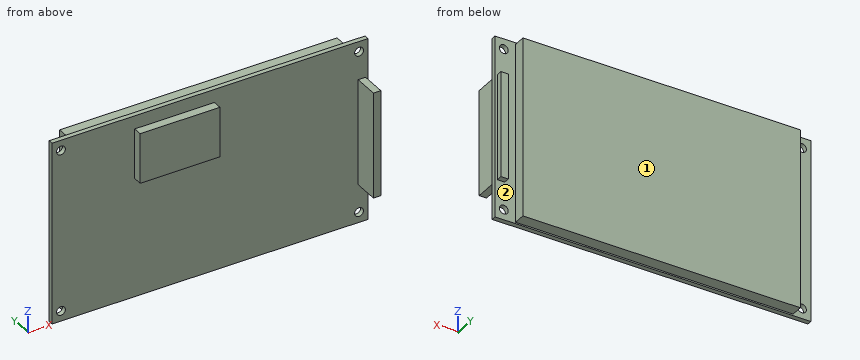
from build123d import *

# Parameters (mm, degrees)
SCHIZZO1_W                        = 94
SCHIZZO1_H                        = 61
ESTRUSIONE_ESTRUSIONE1_DEPTH      = 4
SCHIZZO2_W                        = 107
SCHIZZO2_H                        = 62
ESTRUSIONE_ESTRUSIONE2_DEPTH      = 1.6
ESTRUSIONE_ESTRUSIONE3_DEPTH      = 2
ESTRUSIONE_ESTRUSIONE3_DEPTH_BACK = 10
SCHIZZO4_W                        = 2.5
SCHIZZO4_H                        = 36
SCHIZZO6_R                        = 1.5
TAGLIO_ESTRUSIONE1_DEPTH          = 2
SCHIZZO7_W                        = 27
SCHIZZO7_H                        = 17
ESTRUSIONE_ESTRUSIONE4_DEPTH      = 3


with BuildPart() as part:
    # Schizzo1 → Estrusione-Estrusione1 (new body)
    with BuildSketch(Plane(origin=(0, 0, 0), x_dir=(1, 0, 0), z_dir=(0, 1, 0))):
        Rectangle(SCHIZZO1_W, SCHIZZO1_H)
    extrude(amount=ESTRUSIONE_ESTRUSIONE1_DEPTH)

    # Schizzo2 → Estrusione-Estrusione2 (add)
    with BuildSketch(Plane.XZ):
        with Locations((0.5, 0)):
            Rectangle(SCHIZZO2_W, SCHIZZO2_H)
    extrude(amount=ESTRUSIONE_ESTRUSIONE2_DEPTH)

    # Schizzo4 → Estrusione-Estrusione3 (add, two sides: drawn at the far end of the back side and taken through both)
    with BuildSketch(Plane(origin=(0, 0, 0), x_dir=(1, 0, 0), z_dir=(0, 1, 0)).offset(-ESTRUSIONE_ESTRUSIONE3_DEPTH_BACK)):
        with Locations((51.95, 0)):
            Rectangle(SCHIZZO4_W, SCHIZZO4_H)
    extrude(amount=ESTRUSIONE_ESTRUSIONE3_DEPTH + ESTRUSIONE_ESTRUSIONE3_DEPTH_BACK)

    # Schizzo6 → Taglio-Estrusione1 (cut)
    with BuildSketch(Plane(origin=(0, 0, 0), x_dir=(1, 0, 0), z_dir=(0, 1, 0))):
        with Locations(Location((-50, 27.5, 0), (0, 0, 270))):
            Circle(SCHIZZO6_R)
        with Locations(Location((-50, -27.5, 0), (0, 0, 270))):
            Circle(SCHIZZO6_R)
        with Locations(Location((51, 27.5, 0), (0, 0, 270))):
            Circle(SCHIZZO6_R)
        with Locations(Location((51, -27.5, 0), (0, 0, 270))):
            Circle(SCHIZZO6_R)
    extrude(amount=-TAGLIO_ESTRUSIONE1_DEPTH, mode=Mode.SUBTRACT)

    # Schizzo7 → Estrusione-Estrusione4 (add)
    with BuildSketch(Plane.XZ.offset(1.6)):
        with Locations((-11.5, 18)):
            Rectangle(SCHIZZO7_W, SCHIZZO7_H)
    extrude(amount=ESTRUSIONE_ESTRUSIONE4_DEPTH)


solid = part.part
Design review of the part built by this model. Coordinates are the model's own, in mm. Face numbers are marked on the shaded views. Coordinates: 2 decimals unless noted, no trailing zeros. Loops run counter-clockwise (first coordinate to the right, second up) from the corner with the lowest first, then second, coordinate; pieces in that order, holes last.
Item 1: Add section D-D (z = 13). Write out the cut boundary in (x, y).
Completed:
outline: (-53, -1.6) - (-25, -1.6) - (-25, -4.6) - (2, -4.6) - (2, -1.6) - (50.7, -1.6) - (50.7, -10) - (53.2, -10) - (53.2, -1.6) - (54, -1.6) - (54, 0) - (53.2, 0) - (53.2, 2) - (50.7, 2) - (50.7, 0) - (47, 0) - (47, 4) - (-47, 4) - (-47, 0) - (-53, 0) - close
Item 2: Wall thickness on L1, parallel to X at y = -1.15, z = 27.5; L2, parallel to Y at x = -4.5, z = -6; L3, parallel to X at y = 0.5, z = 8.5: over which ranges is each line inside the solid? List them lowest first.
Completed:
L1: x = -53 to -51.5, -48.5 to 49.5, 52.5 to 54
L2: y = -1.6 to 4
L3: x = -47 to 47, 50.7 to 53.2
Item 3: Add section A-A (x = -50). Write out the cut boundary in (y, z), and give its area (3 significant figures).
Completed:
outline: (-1.6, -31) - (0, -31) - (0, -29) - (-1.6, -29) - close; (-1.6, -26) - (0, -26) - (0, 26) - (-1.6, 26) - close; (-1.6, 29) - (0, 29) - (0, 31) - (-1.6, 31) - close
area: 89.6 mm2
Item 4: Draft analysis for pull direction X (two halves, no side actions). For the marked faces 1 and 2, state which applies: pulls with the +X half, pulls with the -X half, needs draft (parallel to the pull), parting line crosses it, or undercut.
Completed:
face 1: needs draft
face 2: undercut
Item 5: Add section B-B (z = 27.5). Write out the cut boundary in (x, y), and give its area (3 significant figures).
Completed:
outline: (-53, -1.6) - (-51.5, -1.6) - (-51.5, 0) - (-53, 0) - close; (-48.5, -1.6) - (49.5, -1.6) - (49.5, 0) - (47, 0) - (47, 4) - (-47, 4) - (-47, 0) - (-48.5, 0) - close; (52.5, -1.6) - (54, -1.6) - (54, 0) - (52.5, 0) - close
area: 538 mm2
Item 6: Add section C-C (y = -3.5). Write out the cut boundary in (x, z).
Completed:
outline: (-25, 9.5) - (2, 9.5) - (2, 26.5) - (-25, 26.5) - close; (50.7, -18) - (53.2, -18) - (53.2, 18) - (50.7, 18) - close
Item 7: Clearance check with flat-ended pins moving along their axes: pin 1 (0.6 mm diameter, centred on x = 51.5, y = 0.5, fed in from +Z); pin 2 (1.5 mm diameter, centred on x = 3.5, z = -13.5, fed in from -Y); pin 3 (2 mm diameter, centred on x = 52, z = 8, fed in from +Y); pin 4 (2.5 mm diameter, centred on x = -50, z = -27.5, fed in from +Y). State where each tip first meets the part, or that it passes through.
Completed:
pin 1: stops at z = 18
pin 2: stops at y = -1.6
pin 3: stops at y = 2
pin 4: passes through
